from build123d import *

# Parameters (mm, degrees)
SKETCH1_W           = 13.5
SKETCH1_H           = 20
BOSS_EXTRUDE1_DEPTH = 32
SKETCH2_R           = 1.5
CUT_EXTRUDE1_DEPTH  = 41.078048855
SKETCH3_R           = 1.5
CUT_EXTRUDE2_DEPTH  = 41.078048855
SKETCH4_W           = 10
SKETCH4_H           = 22
CUT_EXTRUDE3_DEPTH  = 41.078048855


with BuildPart() as part:
    # Sketch1 → Boss-Extrude1 (new body)
    with BuildSketch(Plane(origin=(0, 0, 0), x_dir=(1, 0, 0), z_dir=(0, 1, 0))):
        with Locations((6.75, -10)):
            Rectangle(SKETCH1_W, SKETCH1_H)
    extrude(amount=BOSS_EXTRUDE1_DEPTH)

    # Sketch2 → Cut-Extrude1 (cut, through all)
    with BuildSketch(Plane.XY.offset(20)):
        with Locations((5, 27)):
            Circle(SKETCH2_R)
        with Locations((5, 5)):
            Circle(SKETCH2_R)
    extrude(amount=-CUT_EXTRUDE1_DEPTH, mode=Mode.SUBTRACT)

    # Sketch3 → Cut-Extrude2 (cut, through all)
    with BuildSketch(Plane(origin=(0, 32, 0), x_dir=(1, 0, 0), z_dir=(0, 1, 0))):
        with Locations(Location((8.5, -10, 0), (0, 0, 270))):
            Circle(SKETCH3_R)
    extrude(amount=-CUT_EXTRUDE2_DEPTH, mode=Mode.SUBTRACT)

    # Sketch4 → Cut-Extrude3 (cut, through all)
    with BuildSketch(Plane(origin=(13.5, 0, 0), x_dir=(0, 0, -1), z_dir=(1, 0, 0))):
        with Locations((-10, 16)):
            Rectangle(SKETCH4_W, SKETCH4_H)
    extrude(amount=-CUT_EXTRUDE3_DEPTH, mode=Mode.SUBTRACT)


solid = part.part
Read the model definition and answer for the solid it produces. Units are mm, in the model's axes. A direction names the side the tool comes from. Coordinates: 2 decimals unless noted, no trailing zeros. Loops run counter-clockwise (first coordinate to the right, second up) from the corner with the lowest first, then second, coordinate; pieces in that order, holes last. Notation, with made-up numbers: (33.5, 22.25) -> (78.5, 22.25) arc R11 ccw to (78.5, 42.25) -> close; hole circle Ø5 at (29.25, -30). An arc over 180 degrees is marked (long way). Write item = value, one per line. Start each with the question number.
1) The part is cut by section D-D, the plane x = 5. Determine the outline of the cut face in (y, z).
2) The part is cut by section A-A, the plane x = 8.5. Determine the outline of the cut face in (y, z), plus the area to 3 significant figures.
3) The mould has two halves that part along Y. Classify faces 1 (the face through (6.7, 0, 9.9)), 2 (the face through (5.69, 3.67, 10.14)), 3 (the face through (13.5, 16, 17)): pulls with the +Y half, pulls with the -Y half, needs draft (parallel to the pull), parting line crosses it, or undercut.
4) For faces 4 (the face through (2, 5, 10)), 5 (the face through (4.805, 28.487, 10.14)), determine the directions among +Z, -Z, +X, -X, +Y, -Y from which every point of the face is accessible in a straight line to the end or side of a thin tool.
5) Find the intervals of material crossed by L1, parallel to X at y = 2.6, z = 10; L2, parallel to Z at x = 11, y = 6.5; L3, parallel to Y at x = 10.5, z = 8.25, in increasing order. Write a range as from..to.
6) Given P1, Ø2, axis at y = 7.5, z = 9.5, coming from the +X side, flat-ended and moving along its own axis, determine where the tip first touches the part or whether it passes through.
7) The part is cut by section C-C, the plane z = 6.5. Determine the outline of the cut face in (x, y).
8) The part is cut by section B-B, the plane y = 20. Determine the outline of the cut face in (x, z).
Result:
q1.outline = (0, 0) -> (3.5, 0) -> (3.5, 20) -> (0, 20) -> close; (6.5, 0) -> (25.5, 0) -> (25.5, 5) -> (6.5, 5) -> close; (6.5, 15) -> (25.5, 15) -> (25.5, 20) -> (6.5, 20) -> close; (28.5, 0) -> (32, 0) -> (32, 20) -> (28.5, 20) -> close
q2.outline = (0, 0) -> (32, 0) -> (32, 8.5) -> (27, 8.5) -> (27, 5) -> (5, 5) -> (5, 8.5) -> (0, 8.5) -> close; (0, 11.5) -> (5, 11.5) -> (5, 15) -> (27, 15) -> (27, 11.5) -> (32, 11.5) -> (32, 20) -> (0, 20) -> close
q2.area = 390 mm²
q3.face_1 = pulls with the -Y half
q3.face_2 = undercut
q3.face_3 = needs draft
q4.face_4 = +X, -X
q4.face_5 = +Z, -Z
q5.L1 = 0..7, 10..13.5
q5.L2 = 0..5, 15..20
q5.L3 = 0..5, 27..32
q6.P1 = through
q7.outline = (0, 0) -> (13.5, 0) -> (13.5, 5) -> (6.5, 5) arc R1.5 cw to (3.5, 5) -> (0, 5) -> close; (0, 27) -> (3.5, 27) arc R1.5 cw to (6.5, 27) -> (13.5, 27) -> (13.5, 32) -> (0, 32) -> close
q8.outline = (0, 0) -> (13.5, 0) -> (13.5, 5) -> (0, 5) -> close; (0, 15) -> (13.5, 15) -> (13.5, 20) -> (0, 20) -> close
